Geometry check sheet. Reference: the model listing, model coordinates, mm. Face numbers are marked on the shaded views. A direction names the side the tool comes from. Give positions to 0.01 mm unless a question says otherwise; leave off trailing zeros. Order: outer loops, then holes, each group sorted by start corner. A loop starts at its lowest first (then second) coordinate and runs counter-clockwise, first axis right, second up. Notation, with made-up numbers: M 76.5,72 L 109.5,72 A19 ccw 109.5,90 Z; hole C 10,-25 d8. An arc over 180 degrees is marked long. Answer as CSV lines item,"result". Start each with the question number.
```python
from build123d import *

# Parameters (mm, degrees)
SKETCH1_R                = 7.5
SKETCH1_R_2              = 8.667102454
BOSS_EXTRUDE1_DEPTH      = 12
SKETCH2_R                = 30
BOSS_EXTRUDE2_DEPTH      = 68
HOLE1_D                  = 30
HOLE1_DEPTH              = 80
HOLE1_CBORE_D            = 40
HOLE1_CBORE_DEPTH        = 16
HOLE1_TIP                = 9.012909285
BOSS_EXTRUDE3_REACH      = 161.452
BOSS_EXTRUDE3_END_RADIUS = 30
CUT_EXTRUDE1_REACH       = 161.452
CUT_EXTRUDE1_END_RADIUS  = 15
SKETCH7_R                = 8


with BuildPart() as part:
    # Sketch1 → Boss-Extrude1 (new body)
    with BuildSketch(Plane(origin=(0, 0, 0), x_dir=(1, 0, 0), z_dir=(0, 1, 0))):
        with BuildLine():
            Line((0, 15), (0, 85))
            ThreePointArc((0, 85), (4.393398282, 95.606601718), (15, 100))
            Line((15, 100), (70.521815275, 100))
            ThreePointArc((70.521815275, 100), (74.404100951, 99.488887394), (78.021815275, 97.990381057))
            Line((78.021815275, 97.990381057), (152.5, 54.990381057))
            ThreePointArc((152.5, 54.990381057), (159.871672921, 43.957892883), (155.606601718, 31.393398282))
            Line((155.606601718, 31.393398282), (128.606601718, 4.393398282))
            ThreePointArc((128.606601718, 4.393398282), (123.740251485, 1.141807012), (118, 0))
            Line((118, 0), (15, 0))
            ThreePointArc((15, 0), (4.393398282, 4.393398282), (0, 15))
        make_face()
        with Locations(Location((15, 85, 0), (0, 0, 270))):
            Circle(SKETCH1_R, mode=Mode.SUBTRACT)
        with Locations(Location((15, 15, 0), (0, 0, 270))):
            Circle(SKETCH1_R_2, mode=Mode.SUBTRACT)
        with Locations(Location((145, 42, 0), (0, 0, 270))):
            Circle(SKETCH1_R, mode=Mode.SUBTRACT)
    extrude(amount=BOSS_EXTRUDE1_DEPTH)

    # Sketch2 → Boss-Extrude2 (add)
    with BuildSketch(Plane(origin=(0, 12, 0), x_dir=(1, 0, 0), z_dir=(0, 1, 0))):
        with Locations(Location((50, 50, 0), (0, 0, 90))):
            Circle(SKETCH2_R)
    extrude(amount=BOSS_EXTRUDE2_DEPTH)

    # Hole1
    with Locations(Plane(origin=(0, 80, 0), x_dir=(1, 0, 0), z_dir=(0, 1, 0))):
        with Locations((50, 50)):
            CounterBoreHole(HOLE1_D / 2, HOLE1_CBORE_D / 2, HOLE1_CBORE_DEPTH, depth=HOLE1_DEPTH)
            with Locations((0, 0, -(HOLE1_DEPTH + HOLE1_TIP / 2))):  # 118° drill point
                Cone(0, HOLE1_D / 2, HOLE1_TIP, mode=Mode.SUBTRACT)

    # Boss-Extrude3: up to this cylinder (the profile starts outside it)
    boss_extrude3_end = Plane(origin=(50, 33.024623, -50), z_dir=(0, -1, 0)) * Cylinder(BOSS_EXTRUDE3_END_RADIUS, 383.904, mode=Mode.PRIVATE)
    # Sketch6 → Boss-Extrude3 (add, up to the surface)
    with BuildSketch(Plane(origin=(95, 0, 0), x_dir=(0, 0, -1), z_dir=(1, 0, 0)), mode=Mode.PRIVATE) as boss_extrude3_sk1:
        with BuildLine():
            Line((35, 42), (35, 12))
            Line((35, 12), (65, 12))
            Line((65, 12), (65, 42))
            ThreePointArc((65, 42), (50, 57), (35, 42))
        make_face()
    boss_extrude3_tool1 = extrude(boss_extrude3_sk1.sketch, amount=-BOSS_EXTRUDE3_REACH, mode=Mode.PRIVATE) - boss_extrude3_end
    add(boss_extrude3_tool1.solids().sort_by_distance((95, 33.024623, -50))[0])

    # Cut-Extrude1: up to this cylinder (the profile starts outside it)
    cut_extrude1_end = Plane(origin=(50, 42, -50), z_dir=(0, 1, 0)) * Cylinder(CUT_EXTRUDE1_END_RADIUS, 353.904, mode=Mode.PRIVATE)
    # Sketch7 → Cut-Extrude1 (cut, up to the surface)
    with BuildSketch(Plane(origin=(95, 0, 0), x_dir=(0, 0, -1), z_dir=(1, 0, 0)), mode=Mode.PRIVATE) as cut_extrude1_sk1:
        with Locations((50, 42)):
            Circle(SKETCH7_R)
    cut_extrude1_tool1 = extrude(cut_extrude1_sk1.sketch, amount=-CUT_EXTRUDE1_REACH, mode=Mode.PRIVATE) - cut_extrude1_end
    add(cut_extrude1_tool1.solids().sort_by_distance((95, 42, -50))[0], mode=Mode.SUBTRACT)


solid = part.part
```
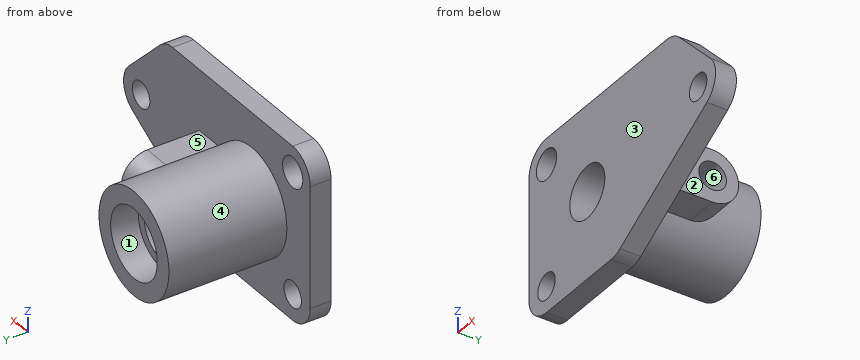
Item 1: Section check A-A on x = 50. Record the boundary of the cut face in (y, z), then the cut area to 3 significant figures.
Item 2: Depth check by flat-ended pin: pin 1 Ø1 at (x, z) = (84.5, -51.5) entering from -Y; pin 2 Ø20 at (x, z) = (48.5, -41.5) entering from +Y; pin 3 Ø17 at (x, z) = (145, -42) entering from +Y; pin 4 Ø24 at (y, z) = (38.5, -48.5) entering from +X. Enter the tip coordinate at first touch or a pass-through.
Item 3: Section check C-C on z = -60. Record the boundary of the cut face in (x, y).
Item 4: Access from +Z, -Z, +X, -X, +Y, -Y to the whole of each face (thin tool, end or side, straight path). Record for the marked faces 4, 5 and 6.
Item 5: Section check D-D on x = 72.5. Record the boundary of the cut face in (y, z), then the cut area to 3 significant figures.
Item 6: Section check B-B on y = 14. Record the boundary of the cut face in (x, z).
Item 7: Scan lines: line 1 along Z through (x, y) = (87.5, 42); line 2 along Y through (x, z) = (78.5, -50); line 3 along Y through (x, z) = (122, -40.5). Record each from-to range of solid material in increasing order.
Item 8: Draft check along X on the marked faces 1, 2 and 3. Enter one of: pulls with the +X half, pulls with the -X half, needs draft (parallel to the pull), parting line crosses it, or undercut.
Numbers:
1,outline,"M 0,-100 L 12,-100 L 12,-80 L 80,-80 L 80,-70 L 64,-70 L 64,-65 L 0,-65 Z; M 0,-35 L 64,-35 L 64,-30 L 80,-30 L 80,-20 L 12,-20 L 12,0 L 0,0 Z"
1,area,"2,720 mm2"
2,pin 1,"y = 0"
2,pin 2,"y = 64"
2,pin 3,"y = 12"
2,pin 4,"x = 95"
3,outline,"M 0,0 L 38.82,0 L 38.82,64 L 32.68,64 L 32.68,80 L 21.72,80 L 21.72,12 L 0,12 Z; M 61.18,0 L 143.82,0 L 143.82,12 L 95,12 L 95,53.18 L 78.28,53.18 L 78.28,80 L 67.32,80 L 67.32,64 L 61.18,64 Z"
4,face 4,"+Y"
4,face 5,"+Z, +X, +Y"
4,face 6,"+X"
5,outline,"M 0,-99.87 L 12,-99.87 L 12,-69.84 L 80,-69.84 L 80,-30.16 L 12,-30.16 L 12,0 L 0,0 Z; hole C 42,-50 d16"
5,area,"3,700 mm2"
6,outline,"M 75.98,-65 L 95,-65 L 95,-35 L 75.98,-35 A30 ccw long Z; hole C 50,-50 d30"
7,line 1,"-65 to -58, -42 to -35"
7,line 2,"0 to 34, 50 to 80"
7,line 3,"0 to 12"
8,face 1,"undercut"
8,face 2,"pulls with the +X half"
8,face 3,"needs draft"
